Read the model definition and answer for the solid it produces. Units are mm, in the model's axes. Face numbers are marked on the shaded views. Coordinates: 2 decimals unless noted, no trailing zeros. Loops run counter-clockwise (first coordinate to the right, second up) from the corner with the lowest first, then second, coordinate; pieces in that order, holes last. Notation, with made-up numbers: (-18.5, 36) - (21.5, 36) arc R21 cw to (21.5, 42) - close; hole circle Ø10 at (-15, 12). An arc over 180 degrees is marked (long way). Use one line per item in the form item = value.
from build123d import *

# Parameters (mm, degrees)
SKETCH2_W           = 52.5507204
SKETCH2_H           = 51.48598542
SKETCH2_W_2         = 3.81
SKETCH2_H_2         = 2.54
BOSS_EXTRUDE1_DEPTH = 5.08
SKETCH3_W           = 47.4707204
SKETCH3_H           = 46.40598542
CUT_EXTRUDE1_DEPTH  = 3.81
SKETCH4_R           = 1.27
CUT_EXTRUDE2_DEPTH  = 3.302
SKETCH5_R           = 5.08
CUT_EXTRUDE3_DEPTH  = 1.9304
SKETCH6_R           = 6.985
BOSS_EXTRUDE2_DEPTH = 38.1
SKETCH8_R           = 5.08
CUT_EXTRUDE4_DEPTH  = 38.1
SKETCH7_W           = 38.1
SKETCH7_H           = 20.32
BOSS_EXTRUDE3_DEPTH = 6.35
FILLET3_R           = 2.54
SKETCH9_W           = 6.35
SKETCH9_H           = 3.81
CUT_EXTRUDE5_DEPTH  = 11.938


with BuildPart() as part:
    # Sketch2 → Boss-Extrude1 (new body)
    with BuildSketch(Plane(origin=(0, 0, 0), x_dir=(1, 0, 0), z_dir=(0, 1, 0))):
        with Locations((0, 3.81e-06)):
            Rectangle(SKETCH2_W, SKETCH2_H)
        with Locations((28.1803602, 1.27)):
            Rectangle(SKETCH2_W_2, SKETCH2_H_2)
        with Locations((-28.1803602, 1.2700127)):
            Rectangle(SKETCH2_W_2, SKETCH2_H_2)
    extrude(amount=BOSS_EXTRUDE1_DEPTH)

    # Sketch3 → Cut-Extrude1 (cut)
    with BuildSketch(Plane.XZ):
        with Locations((0, -3.81e-06)):
            Rectangle(SKETCH3_W, SKETCH3_H)
    extrude(amount=-CUT_EXTRUDE1_DEPTH, mode=Mode.SUBTRACT)

    # Sketch4 → Cut-Extrude2 (cut)
    with BuildSketch(Plane.XY):
        with Locations((28.1803602, 2.54)):
            Circle(SKETCH4_R)
        with Locations((-28.1803602, 2.54)):
            Circle(SKETCH4_R)
    extrude(amount=-CUT_EXTRUDE2_DEPTH, mode=Mode.SUBTRACT)

    # Sketch5 → Cut-Extrude3 (cut)
    with BuildSketch(Plane(origin=(0, 5.08, 0), x_dir=(1, 0, 0), z_dir=(0, 1, 0))):
        Circle(SKETCH5_R)
    extrude(amount=-CUT_EXTRUDE3_DEPTH, mode=Mode.SUBTRACT)

    # Sketch6 → Boss-Extrude2 (add)
    with BuildSketch(Plane(origin=(0, 5.08, 0), x_dir=(1, 0, 0), z_dir=(0, 1, 0))):
        Circle(SKETCH6_R)
    extrude(amount=BOSS_EXTRUDE2_DEPTH)

    # Sketch8 → Cut-Extrude4 (cut)
    with BuildSketch(Plane(origin=(0, 43.18, 0), x_dir=(1, 0, 0), z_dir=(0, 1, 0))):
        Circle(SKETCH8_R)
    extrude(amount=-CUT_EXTRUDE4_DEPTH, mode=Mode.SUBTRACT)

    # Sketch7 → Boss-Extrude3 (add)
    with BuildSketch(Plane(origin=(0, 43.18, 0), x_dir=(1, 0, 0), z_dir=(0, 1, 0))):
        Rectangle(SKETCH7_W, SKETCH7_H)
    extrude(amount=BOSS_EXTRUDE3_DEPTH)

    # Fillet3
    fillet3_edges = [part.edges().sort_by_distance(p)[0] for p in [
        (-19.05, 43.18, 0),
        (0, 43.18, 10.16),
        (19.05, 43.18, 0),
        (0, 43.18, -10.16),
    ]]
    fillet(fillet3_edges, radius=FILLET3_R)

    # Sketch9 → Cut-Extrude5 (cut)
    with BuildSketch(Plane.XY.offset(0.3429889)):
        with Locations((0, 32.385)):
            Rectangle(SKETCH9_W, SKETCH9_H)
    extrude(amount=CUT_EXTRUDE5_DEPTH, mode=Mode.SUBTRACT)


solid = part.part
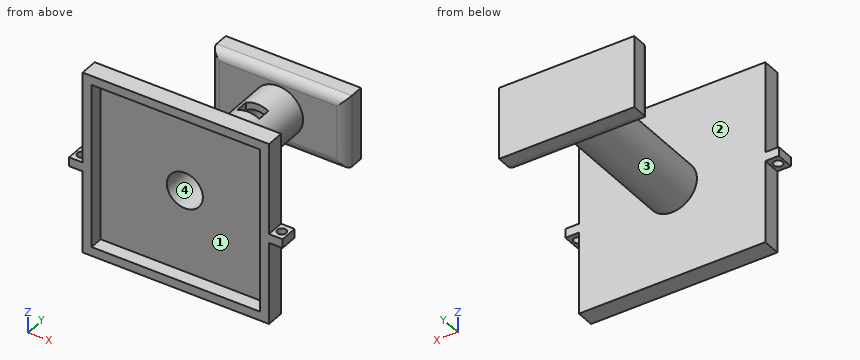
Item 1: The part is cut by section C-C on x = -20.5. Give the vertices of the cut face in (y, z), plus the area to 3 significant figures.
Results below:
outline = (0, -25.74) - (5.08, -25.74) - (5.08, 25.74) - (0, 25.74) - (0, 23.2) - (3.81, 23.2) - (3.81, -23.2) - (0, -23.2) - close
area = 84.7 mm²
Item 2: Each of these flat-tipped pins is pushed along its axis until it touches: P1, Ø4, axis at x = -28, y = 2, coming from the -Z side; P2, Ø6, axis at x = 0, z = 0, coming from the -Y side; P3, Ø2.5, axis at y = 3.5, z = 13, coming from the +X side; P4, Ø3, axis at x = 9, y = 48.5, coming from the -Z side. Where does it stop, or does it pass through?
Results below:
P1 = -25.74
P2 = 43.18
P3 = 26.28
P4 = -10.16
Item 3: For a pull along Y with two mould halves and no side action, classify the marked faces 1, 2, 3 and 4 as +Y half, -Y half, draft (parallel to the pull), parting line (faces both ways), or undercut.
Results below:
face_1 = -Y half
face_2 = undercut
face_3 = undercut
face_4 = draft
Item 4: The part is cut by section A-A on y = 2.54. Give the vertices of the cut face in (x, z).
Results below:
outline = (-30.09, -2.54) - (-29.45, -2.54) - (-29.45, 0) - (-30.09, 0) - close; (-26.91, -2.54) - (-26.28, -2.54) - (-26.28, -25.74) - (26.28, -25.74) - (26.28, -2.54) - (26.91, -2.54) - (26.91, 0) - (26.28, 0) - (26.28, 25.74) - (-26.28, 25.74) - (-26.28, 0) - (-26.91, 0) - close; (29.45, -2.54) - (30.09, -2.54) - (30.09, 0) - (29.45, 0) - close; hole (-23.74, -23.2) - (23.74, -23.2) - (23.74, 23.2) - (-23.74, 23.2) - close
Item 5: Find the intervals of material crossed by L1, parallel to X at y = 23.5, z = 0 (3 decimals); L2, parallel to Y at x = -17.5, z = 0.5; L3, parallel to Y at x = -26, z = -23.5, in increasing order.
Results below:
L1 = -6.985 to -5.08, 5.08 to 6.985
L2 = 3.81 to 5.08, 43.38 to 49.53
L3 = 0 to 5.08
Item 6: The part is cut by section D-D on z = 18.5. Give the vertices of the cut face in (x, y), plus the area to 3 significant figures.
Results below:
outline = (-26.28, 0) - (-23.74, 0) - (-23.74, 3.81) - (23.74, 3.81) - (23.74, 0) - (26.28, 0) - (26.28, 5.08) - (-26.28, 5.08) - close
area = 86.1 mm²
Item 7: The part is cut by section B-B on x = 14. Give the vertices of the cut face in (y, z), plus the area to 3 significant figures.
Results below:
outline = (0, -25.74) - (5.08, -25.74) - (5.08, 25.74) - (0, 25.74) - (0, 23.2) - (3.81, 23.2) - (3.81, -23.2) - (0, -23.2) - close; (43.18, -7.62) arc R2.54 ccw to (45.72, -10.16) - (49.53, -10.16) - (49.53, 10.16) - (45.72, 10.16) arc R2.54 ccw to (43.18, 7.62) - close
area = 211 mm²
